Could you check a few things on this model? Use its own coordinates, in mm. Coordinates: 2 decimals unless noted, no trailing zeros. Write each loop counter-clockwise with the first axis right and the second up, starting at its lowest first coordinate (ties: lowest second). Pieces come first, ordered by that corner, then holes.
Item 1: I want a section at A-A on x = 67.31. Please give me the cut outline in (y, z), then the cut area to 3 significant figures.
Item 2: I want a section at C-C on y = -3.6. State how many separate pieces and enclosed holes the cut face has, then the cut area to 3 significant figures.
Item 3: If I drill on probe 1 along X at (y, z) = (-4.4, 45.5); probe 2 along Z at (x, y) = (41, -3.25); probe 3 along Z at (x, y) = (-32, -3.15), over which ranges is the centre line in solid material (lowest first)?
Item 4: For P1, Ø1.5, axis at y = -1, z = 0, coming from the -X side; P2, Ø1, axis at x = 12.67, z = 15.89, coming from the +Y side; P3, Ø1, axis at x = -29, y = -2.5, coming from the +Z side, each with a flat end and sliding along its axis, tell me the tip position at first contact or that it passes through.
Item 5: I want a section at B-B on z = -38.1. Please give me the cut outline in (x, y) (3 decimals).
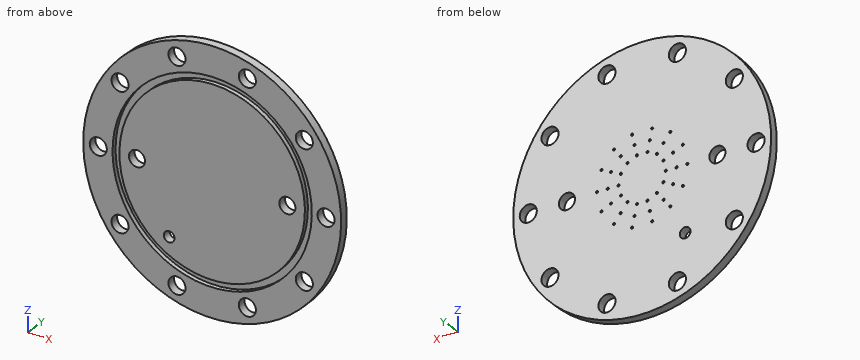
from build123d import *

# Parameters (mm, degrees)
F_3_8_CLEARANCE_HOLE1_D      = 10.0838
CIRPATTERN1_COUNT            = 10
F_3_8_0_375_DIAMETER_HOLE1_D = 9.525
F_1_4_0_25_DIAMETER_HOLE1_D  = 6.35
SKETCH7_R                    = 0.635
CUT_EXTRUDE1_DEPTH           = 2.54


with BuildPart() as part:
    # Sketch1 → Revolve1 (revolve)
    with BuildSketch(Plane.XY, mode=Mode.PRIVATE) as revolve1_sk:
        Polygon((0, 0), (0, -5.08), (54.8259, -5.08), (54.8259, -2.3876), (58.8899, -2.3876), (58.8899, -5.08), (76.2, -5.08), (76.2, 0), align=None)
    revolve(revolve1_sk.sketch.rotate(Axis((0, 0, 0), (0, -1, 0)), 90), axis=Axis((0, 0, 0), (0, -1, 0)))

    # 3_8 Clearance Hole1 (through all)
    with Locations(Plane(origin=(67.31, 0, 0), x_dir=(0, 0, 1), z_dir=(0, 1, 0))):
        with Locations((0, 0)):
            f_3_8_clearance_hole1 = Hole(F_3_8_CLEARANCE_HOLE1_D / 2)

    # CirPattern1: 3_8 Clearance Hole1 ×10 about axis
    cirpattern1_axis = Axis((0, 0, 0), (0, 1, 0))
    for i in range(1, CIRPATTERN1_COUNT):
        add(f_3_8_clearance_hole1.rotate(cirpattern1_axis, i * 360 / CIRPATTERN1_COUNT), mode=Mode.SUBTRACT)

    # 3_8 _0.375_ Diameter Hole1 (through all)
    with Locations(Plane(origin=(44.45, 0, 0), x_dir=(0, 0, 1), z_dir=(0, 1, 0))):
        with Locations((0, 0), (0, -88.9)):
            Hole(F_3_8_0_375_DIAMETER_HOLE1_D / 2)

    # 1_4 _0.25_ Diameter Hole1 (through all)
    with Locations(Plane(origin=(-25.4, 0, -38.1), x_dir=(0, 0, 1), z_dir=(0, 1, 0))):
        with Locations((0, 0)):
            Hole(F_1_4_0_25_DIAMETER_HOLE1_D / 2)

    # Sketch7 → Cut-Extrude1 (cut)
    with BuildSketch(Plane(origin=(0, 0, 0), x_dir=(1, 0, 0), z_dir=(0, 1, 0))):
        with Locations(Location((13.97, 0, 0), (0, 0, 270))):
            Circle(SKETCH7_R)
        with Locations(Location((20.32, 0, 0), (0, 0, 270))):
            Circle(SKETCH7_R)
        with Locations(Location((26.67, 0, 0), (0, 0, 270))):
            Circle(SKETCH7_R)
        with Locations(Location((12.586535085, -6.061355835, 0), (0, 0, 270))):
            Circle(SKETCH7_R)
        with Locations(Location((18.307687396, -8.816517579, 0), (0, 0, 270))):
            Circle(SKETCH7_R)
        with Locations(Location((24.028839707, -11.571679322, 0), (0, 0, 270))):
            Circle(SKETCH7_R)
        with Locations(Location((8.710152532, -10.92218581, 0), (0, 0, 270))):
            Circle(SKETCH7_R)
        with Locations(Location((12.669312774, -15.886815724, 0), (0, 0, 270))):
            Circle(SKETCH7_R)
        with Locations(Location((16.628473016, -20.851445637, 0), (0, 0, 270))):
            Circle(SKETCH7_R)
        with Locations(Location((3.108617447, -13.619742933, 0), (0, 0, 270))):
            Circle(SKETCH7_R)
        with Locations(Location((4.521625378, -19.810535176, 0), (0, 0, 270))):
            Circle(SKETCH7_R)
        with Locations(Location((5.934633309, -26.001327418, 0), (0, 0, 270))):
            Circle(SKETCH7_R)
        with Locations(Location((-3.108617447, -13.619742933, 0), (0, 0, 270))):
            Circle(SKETCH7_R)
        with Locations(Location((-4.521625378, -19.810535176, 0), (0, 0, 270))):
            Circle(SKETCH7_R)
        with Locations(Location((-5.934633309, -26.001327418, 0), (0, 0, 270))):
            Circle(SKETCH7_R)
        with Locations(Location((-8.710152532, -10.92218581, 0), (0, 0, 270))):
            Circle(SKETCH7_R)
        with Locations(Location((-12.669312774, -15.886815724, 0), (0, 0, 270))):
            Circle(SKETCH7_R)
        with Locations(Location((-16.628473016, -20.851445637, 0), (0, 0, 270))):
            Circle(SKETCH7_R)
        with Locations(Location((-12.586535085, -6.061355835, 0), (0, 0, 270))):
            Circle(SKETCH7_R)
        with Locations(Location((-18.307687396, -8.816517579, 0), (0, 0, 270))):
            Circle(SKETCH7_R)
        with Locations(Location((-24.028839707, -11.571679322, 0), (0, 0, 270))):
            Circle(SKETCH7_R)
        with Locations(Location((-13.97, 0, 0), (0, 0, 270))):
            Circle(SKETCH7_R)
        with Locations(Location((-20.32, 0, 0), (0, 0, 270))):
            Circle(SKETCH7_R)
        with Locations(Location((-26.67, 0, 0), (0, 0, 270))):
            Circle(SKETCH7_R)
        with Locations(Location((-12.586535085, 6.061355835, 0), (0, 0, 270))):
            Circle(SKETCH7_R)
        with Locations(Location((-18.307687396, 8.816517579, 0), (0, 0, 270))):
            Circle(SKETCH7_R)
        with Locations(Location((-24.028839707, 11.571679322, 0), (0, 0, 270))):
            Circle(SKETCH7_R)
        with Locations(Location((-8.710152532, 10.92218581, 0), (0, 0, 270))):
            Circle(SKETCH7_R)
        with Locations(Location((-12.669312774, 15.886815724, 0), (0, 0, 270))):
            Circle(SKETCH7_R)
        with Locations(Location((-16.628473016, 20.851445637, 0), (0, 0, 270))):
            Circle(SKETCH7_R)
        with Locations(Location((-3.108617447, 13.619742933, 0), (0, 0, 270))):
            Circle(SKETCH7_R)
        with Locations(Location((-4.521625378, 19.810535176, 0), (0, 0, 270))):
            Circle(SKETCH7_R)
        with Locations(Location((-5.934633309, 26.001327418, 0), (0, 0, 270))):
            Circle(SKETCH7_R)
        with Locations(Location((3.108617447, 13.619742933, 0), (0, 0, 270))):
            Circle(SKETCH7_R)
        with Locations(Location((4.521625378, 19.810535176, 0), (0, 0, 270))):
            Circle(SKETCH7_R)
        with Locations(Location((5.934633309, 26.001327418, 0), (0, 0, 270))):
            Circle(SKETCH7_R)
        with Locations(Location((8.710152532, 10.92218581, 0), (0, 0, 270))):
            Circle(SKETCH7_R)
        with Locations(Location((12.669312774, 15.886815724, 0), (0, 0, 270))):
            Circle(SKETCH7_R)
        with Locations(Location((16.628473016, 20.851445637, 0), (0, 0, 270))):
            Circle(SKETCH7_R)
        with Locations(Location((12.586535085, 6.061355835, 0), (0, 0, 270))):
            Circle(SKETCH7_R)
        with Locations(Location((18.307687396, 8.816517579, 0), (0, 0, 270))):
            Circle(SKETCH7_R)
        with Locations(Location((24.028839707, 11.571679322, 0), (0, 0, 270))):
            Circle(SKETCH7_R)
    extrude(amount=-CUT_EXTRUDE1_DEPTH, mode=Mode.SUBTRACT)


solid = part.part
Response values:
1. outline: (-5.08, -35.72) - (0, -35.72) - (0, -5.04) - (-5.08, -5.04) - close; (-5.08, 5.04) - (0, 5.04) - (0, 35.72) - (-5.08, 35.72) - close
1. area: 312 mm2
2. separate pieces: 2
2. enclosed holes: 14
2. area: 15,800 mm2
3. probe 1: x = -61.12 to -37.39, -30.59 to 30.59, 37.39 to 61.12
3. probe 2: z = -64.23 to -42.27, -36.4 to -3.28, 3.28 to 36.4, 42.27 to 64.23
3. probe 3: z = -69.16 to -49.44, -44.52 to 44.52, 49.44 to 69.16
4. P1: stops at x = -76.2
4. P2: stops at y = -2.54
4. P3: stops at z = 70.67
5. outline: (-65.991, -5.08) - (-59.28, -5.08) - (-59.28, 0) - (-65.991, 0) - close; (-49.63, -5.08) - (-44.904, -5.08) - (-44.904, -2.388) - (-39.424, -2.388) - (-39.424, -5.08) - (-28.575, -5.08) - (-28.575, 0) - (-49.63, 0) - close; (-22.225, -5.08) - (39.424, -5.08) - (39.424, -2.388) - (44.904, -2.388) - (44.904, -5.08) - (49.63, -5.08) - (49.63, 0) - (-22.225, 0) - close; (59.28, -5.08) - (65.991, -5.08) - (65.991, 0) - (59.28, 0) - close
